For this review, take the finished solid that the model builds, in its own axes (mm). A direction names the side the tool comes from. Round coordinates to 2 decimals unless told otherwise and drop trailing zeros. Write each loop counter-clockwise with the first axis right and the second up, starting at its lowest first coordinate (ties: lowest second). Pieces come first, ordered by that corner, then holes. Notation, with made-up numbers: M -23,25 L -1,25 A12 ccw -1,47 Z; hole C 26,16 d10. An arc over 180 degrees is marked long. Use one line per item in the form item = value. Start each with the question number.
Item 1: For faces 5 (the cylindrical face through (23.54, 1.565, 598.366)), 6 (the flat face through (26, 22.225, 301)), 7 (the cylindrical face through (14.87, 23.835, 15.744)), list the 3-axis set-ups (+Z, -Z, +X, -X, +Y, -Y) from which the entire face can be reached by the end or side of a thin tool; tool diameter is ignored.
Item 2: For line 1 (Z direction, x = 25.4, y = 23.1); line 2 (Z direction, x = 25.4, y = 2.45); line 3 (X direction, y = 6, z = 564) (3 decimals), list the stretches that pass through material, from the lowest coordinate up. Write a range as [from, to].
Item 3: Add section B-B (y = 17.5). State the section outline as (x, z) points (3 decimals), and give its area (3 significant figures).
Item 4: Add section C-C (z = 106.5). State the section outline as (x, y) points (3 decimals), and give its area (3 significant figures).
Item 5: Add section D-D (z = 584.2). State the section outline as (x, y) points (1 decimal), and give its area (3 significant figures).
Item 6: Add section A-A (z = 25.4). State the section outline as (x, y) points (1 decimal), and give its area (3 significant figures).
Item 7: Draft analysis for pull direction Y (two halves, no side actions). For faces 1 (the flat face through (25, 0, 301)), 2 (the flat face through (25, 25.4, 301)), 3 (the flat face through (26, 3.175, 301)), 4 (the cylindrical face through (24.78, 23.83, 554.08)), state which applies: released by +Y, released by -Y, zero draft, split by the parting line, or undercut.
from build123d import *

# Parameters (mm, degrees)
SKETCH1_W           = 50.8
SKETCH1_H           = 25.4
BOSS_EXTRUDE1_DEPTH = 609.6
SKETCH2_W           = 44.45
SKETCH2_H           = 19.05
CUT_EXTRUDE1_DEPTH  = 635
SKETCH6_R           = 14.2875
CUT_EXTRUDE5_DEPTH  = 25.4
SKETCH7_R           = 14.2875
CUT_EXTRUDE6_DEPTH  = 3.175
SKETCH8_R           = 4.7625
CUT_EXTRUDE7_DEPTH  = 25.4


with BuildPart() as part:
    # Sketch1 → Boss-Extrude1 (new body)
    with BuildSketch(Plane.XY):
        with Locations((25.4, 12.7)):
            Rectangle(SKETCH1_W, SKETCH1_H)
    extrude(amount=BOSS_EXTRUDE1_DEPTH)

    # Sketch2 → Cut-Extrude1 (cut)
    with BuildSketch(Plane(origin=(0, 0, 0), x_dir=(-1, 0, 0), z_dir=(0, 0, -1))):
        with Locations((-25.4, 12.7)):
            Rectangle(SKETCH2_W, SKETCH2_H)
    extrude(amount=-CUT_EXTRUDE1_DEPTH, mode=Mode.SUBTRACT)

    # Sketch6 → Cut-Extrude5 (cut)
    with BuildSketch(Plane(origin=(0, 25.4, 0), x_dir=(1, 0, 0), z_dir=(0, 1, 0))):
        with Locations((25.4, -25.4)):
            Circle(SKETCH6_R)
    extrude(amount=-CUT_EXTRUDE5_DEPTH, mode=Mode.SUBTRACT)

    # Sketch7 → Cut-Extrude6 (cut)
    with BuildSketch(Plane.XZ):
        with Locations((25.4, 584.2)):
            Circle(SKETCH7_R)
    extrude(amount=-CUT_EXTRUDE6_DEPTH, mode=Mode.SUBTRACT)

    # Sketch8 → Cut-Extrude7 (cut)
    with BuildSketch(Plane(origin=(0, 25.4, 0), x_dir=(1, 0, 0), z_dir=(0, 1, 0))):
        with Locations((25.4, -558.8)):
            Circle(SKETCH8_R)
    extrude(amount=-CUT_EXTRUDE7_DEPTH, mode=Mode.SUBTRACT)


solid = part.part
Calculated:
q1.face_5 = -Y
q1.face_6 = +Z, -Z
q1.face_7 = +Y, -Y
q2.line_1 = [0, 11.11], [39.69, 554.04], [563.56, 609.6]
q2.line_2 = [0, 11.11], [39.69, 554.04], [563.56, 569.91], [598.49, 609.6]
q2.line_3 = [0, 3.175], [47.625, 50.8]
q3.outline = M 0,0 L 3.175,0 L 3.175,609.6 L 0,609.6 Z; M 47.625,0 L 50.8,0 L 50.8,609.6 L 47.625,609.6 Z
q3.area = 3,870 mm^2
q4.outline = M 0,0 L 50.8,0 L 50.8,25.4 L 0,25.4 Z; hole M 3.175,3.175 L 47.625,3.175 L 47.625,22.225 L 3.175,22.225 Z
q4.area = 444 mm^2
q5.outline = M 0,0 L 11.1,0 L 11.1,3.2 L 3.2,3.2 L 3.2,22.2 L 47.6,22.2 L 47.6,3.2 L 39.7,3.2 L 39.7,0 L 50.8,0 L 50.8,25.4 L 0,25.4 Z
q5.area = 353 mm^2
q6.outline = M 0,0 L 11.1,0 L 11.1,3.2 L 3.2,3.2 L 3.2,22.2 L 11.1,22.2 L 11.1,25.4 L 0,25.4 Z; M 39.7,0 L 50.8,0 L 50.8,25.4 L 39.7,25.4 L 39.7,22.2 L 47.6,22.2 L 47.6,3.2 L 39.7,3.2 Z
q6.area = 262 mm^2
q7.face_1 = released by -Y
q7.face_2 = released by +Y
q7.face_3 = undercut
q7.face_4 = zero draft
